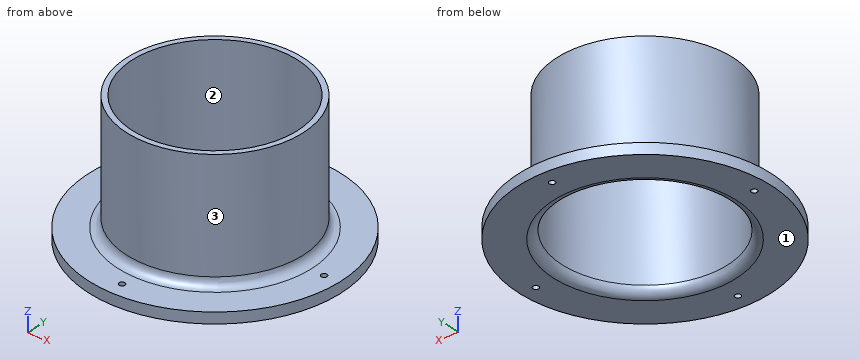
```python
from build123d import *

# Parameters (mm, degrees)
F0_R     = 51.59375
F1_DEPTH = 76.2
F2_R     = 73.81875
F3_DEPTH = 6.35
F4_R     = 48.41875
F5_DEPTH = 76.201
F6_R     = 5.08
F7_R     = 5.08
F8_R     = 1.732497
F9_DEPTH = 6.351


with BuildPart() as f1:
    # F0 (on Top) → F1 (new body)
    with BuildSketch(Plane.XY):
        Circle(F0_R)
    extrude(amount=F1_DEPTH)

    # F2 (on Top) → F3 (join)
    with BuildSketch(Plane.XY):
        Circle(F2_R)
    extrude(amount=F3_DEPTH)

    # F4 (on face) → F5 (cut, through all)
    with BuildSketch(Plane.XY.offset(76.2)):
        Circle(F4_R)
    extrude(amount=-F5_DEPTH, mode=Mode.SUBTRACT)

    # F6
    f6_edges = [f1.edges().sort_by_distance(p)[0] for p in [
        (-51.59375, 0, 6.35),
    ]]
    fillet(f6_edges, radius=F6_R)

    # F7
    f7_edges = [f1.edges().sort_by_distance(p)[0] for p in [
        (-48.41875, 0, 0),
    ]]
    fillet(f7_edges, radius=F7_R)

    # F8 (on face) → F9 (cut, through all)
    with BuildSketch(Plane.XY.offset(6.35)):
        with Locations((64.809114, 0)):
            Circle(F8_R)
        with Locations((0, 64.809114)):
            Circle(F8_R)
        with Locations((-64.809114, 0)):
            Circle(F8_R)
        with Locations((0, -64.809114)):
            Circle(F8_R)
    extrude(amount=-F9_DEPTH, mode=Mode.SUBTRACT)


solid = f1.part
```
Geometry: final body of the model. Coordinates: model frame, mm. Face numbers are marked on the shaded views. Give positions to 0.01 mm unless a question says otherwise; leave off trailing zeros. Write each loop counter-clockwise with the first axis right and the second up, starting at its lowest first coordinate (ties: lowest second). Pieces come first, ordered by that corner, then holes.
1. Pin query (flat end, axial travel): P1, Ø5, axis at x = -5.5, z = 47, coming from the +Y side; P2, Ø3, axis at x = 0, y = -64.81, coming from the +Z side; P3, Ø5, axis at y = 27.5, z = 64.5, coming from the +X side; P4, Ø2, axis at x = -18.5, z = 22, coming from the -Y side. Return the tip coordinate at first contact, or that it passes through.
2. Line query: probe 1 along Y at (x, z) = (0, 4); probe 2 along Y at (x, z) = (0, 3.5); probe 3 along Z at (x, y) = (-27.5, -63). Output: solid intervals per line, ascending.
3. Draft query along Y for the marked faces 1, 2 and 3. Return one class per face: released by +Y, released by -Y, zero draft, split by the parting line, or undercut.
4. Section query A-A, the plane z = 52. Return loops of the section in (x, y), then the cut area to 3 significant figures.
Computed:
1. P1: stops at y = 51.51
1. P2: passes through
1. P3: stops at x = 45.13
1. P4: stops at y = -48.54
2. probe 1: y = -73.82 to -66.54, -63.08 to -48.53, 48.53 to 63.08, 66.54 to 73.82
2. probe 2: y = -73.82 to -66.54, -63.08 to -48.67, 48.67 to 63.08, 66.54 to 73.82
2. probe 3: z = 0 to 6.35
3. face 1: zero draft
3. face 2: undercut
3. face 3: split by the parting line
4. outline: circle Ø103.19 at (0, 0); hole circle Ø96.84 at (0, 0)
4. area: 998 mm2
